Check sheet for the drawn part. Datum: minimum x, y, z corner. Units: mm. A direction names the side the tool comes from. Round coordinates to 2 decimals unless told otherwise and drop trailing zeros. Order: outer loops, then holes, each group sorted by start corner. A loop starts at its lowest first (then second) coordinate and runs counter-clockwise, first axis right, second up. Notation, with made-up numbers: M -13,37 L 0,37 A20 ccw 0,55 Z; hole C 21,64 d4. An arc over 180 degrees is marked long. Use one line per item in the form item = value. Start each with the question number.
Item 1: Thickness scan on probe 1 along Y at (x, z) = (2, 0.6); probe 2 along Z at (x, y) = (17.25, 15.5); probe 3 along Z at (x, y) = (23.75, 13.5). Record the ranges inside material, lowest first. Write a range as [from, to].
Item 2: Cross-section at B-B on x = 23. Enter the section's corners in (y, z).
Item 3: Cross-section at C-C on y = 2. Enter the section's corners in (x, z), then the cut area to 3 significant figures.
Item 4: Cross-section at D-D on z = 3. Enter the section's corners in (x, y), then the cut area to 3 significant figures.
Item 5: Cross-section at A-A on y = 14.5. Enter the section's corners in (x, z).
Item 6: Go/stop test with flat-tipped pins: pin 1 Ø2 at (y, z) = (14, 3) entering from -X; pin 2 Ø2 at (x, z) = (10, 3.5) entering from +Y; pin 3 Ø3 at (x, y) = (2, 2) entering from +Z. Record where each tip stops, or that it passes through.
Item 7: Tool access check on the marked faces 1, 2 and 3. Record the directions out of +Z, -Z, +X, -X, +Y, -Y that give a thin tool (end or side, any length) a straight path to the whole face; none if there is none.
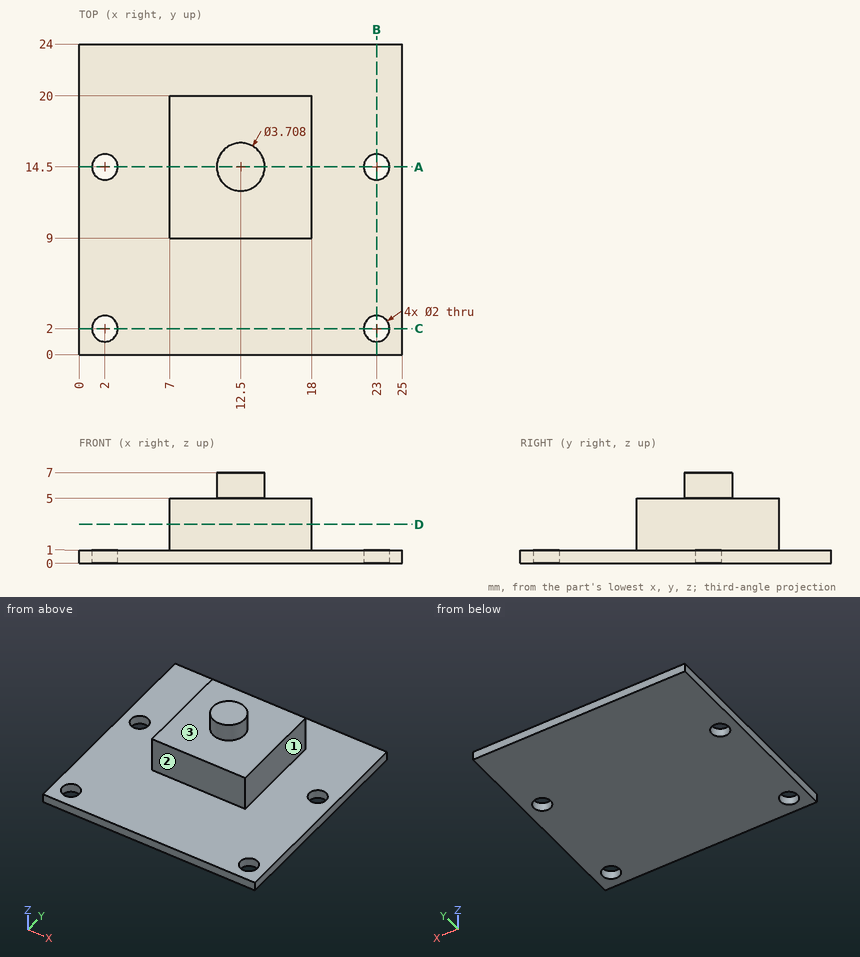
Output values:
q1.probe_1 = [0, 1], [3, 13.5], [15.5, 24]
q1.probe_2 = [0, 5]
q1.probe_3 = [0, 1]
q2.outline = M 0,0 L 1,0 L 1,1 L 0,1 Z; M 3,0 L 13.5,0 L 13.5,1 L 3,1 Z; M 15.5,0 L 24,0 L 24,1 L 15.5,1 Z
q3.outline = M 0,0 L 1,0 L 1,1 L 0,1 Z; M 3,0 L 22,0 L 22,1 L 3,1 Z; M 24,0 L 25,0 L 25,1 L 24,1 Z
q3.area = 21.0 mm2
q4.outline = M 7,9 L 18,9 L 18,20 L 7,20 Z
q4.area = 121 mm2
q5.outline = M 0,0 L 1,0 L 1,1 L 0,1 Z; M 3,0 L 22,0 L 22,1 L 18,1 L 18,5 L 14.35,5 L 14.35,7 L 10.65,7 L 10.65,5 L 7,5 L 7,1 L 3,1 Z; M 24,0 L 25,0 L 25,1 L 24,1 Z
q6.pin_1 = 7
q6.pin_2 = 20
q6.pin_3 = 1
q7.face_1 = +Z, +X, +Y, -Y
q7.face_2 = +Z, +X, -X, -Y
q7.face_3 = +Z
